Autodesk Inventor part; units mm, degrees
ref_plane "YZ Plane" through (0, 0, 0) normal (1, 0, 0) x (0, 1, 0)
ref_plane "XZ Plane" through (0, 0, 0) normal (0, 1, 0) x (-1, 0, 0)
ref_plane "XY Plane" through (0, 0, 0) normal (0, 0, 1) x (1, 0, 0)
sketch "Sketch1" plane through (0, 0, 0) normal (0, 0, 1) x (1, 0, 0)
  arc A0 (-220.016275, 220.016275) -> (-311.15, 0) centre (0, 0) ccw
  line L0 (-311.15, 0) -> (-304.8, 0)
  line L1 (0, 0) -> (-220.016275, 220.016275)
  line L2 (-311.15, 0) -> (0, 0)
extrude "Extrusion1" add sketch "Sketch1" along normal blind 3.175
sketch "Sketch4" plane through (0, 0, 0) normal (0, 0, -1) x (-1, 0, 0)
  arc A0 (311.15, 0) -> (220.016275, 220.016275) centre (0, 0) ccw
  line L0 (220.016275, 220.016275) -> (0, 0)
  line L1 (0, 0) -> (311.15, 0)
  arc A1 (301.625, 0) -> (213.281083, 213.281083) centre (0, 0) ccw
  arc A2 (303.2125, 0) -> (214.403615, 214.403615) centre (0, 0) ccw
  arc A3 (304.8, 0) -> (215.526147, 215.526147) centre (0, 0) ccw construction
  arc A4 (300.0375, 0) -> (212.158551, 212.158551) centre (0, 0) ccw construction
  circle A5 centre (215.526147, 215.526147) radius 1.5875
  circle A6 centre (212.158551, 212.158551) radius 1.5875
  circle A7 centre (233.490346, 195.921663) radius 1.5875
  circle A8 centre (229.84206, 192.860387) radius 1.5875
  circle A9 centre (249.677543, 174.826098) radius 1.5875
  circle A10 centre (245.776331, 172.09444) radius 1.5875
  circle A11 centre (263.964543, 152.4) radius 1.5875
  circle A12 centre (259.840097, 150.01875) radius 1.5875
  circle A13 centre (276.242613, 128.814046) radius 1.5875
  circle A14 centre (271.926323, 126.801327) radius 1.5875
  circle A15 centre (286.418311, 104.24774) radius 1.5875
  circle A16 centre (281.943025, 102.618869) radius 1.5875
  circle A17 centre (294.414192, 78.888045) radius 1.5875
  circle A18 centre (289.81397, 77.655419) radius 1.5875
  circle A19 centre (300.169403, 52.927965) radius 1.5875
  circle A20 centre (295.479256, 52.100965) radius 1.5875
  circle A21 centre (303.640144, 26.56507) radius 1.5875
  circle A22 centre (298.895767, 26.149991) radius 1.5875
  circle A23 centre (304.8, 0) radius 1.5875
  circle A24 centre (300.0375, 0) radius 1.5875
  circle A25 centre (219.969498, 210.989242) radius 1.5875
  circle A26 centre (304.733847, 6.35) radius 1.5875
  point P0 (231.058155, 193.880813)
  point P1 (232.274251, 194.901238)
  point P2 (247.076735, 173.004993)
  point P3 (248.377139, 173.915545)
  point P4 (261.214912, 150.8125)
  point P5 (262.589728, 151.60625)
  point P6 (273.365086, 127.472233)
  point P7 (274.80385, 128.14314)
  point P8 (283.434787, 103.161826)
  point P9 (284.926549, 103.704783)
  point P10 (291.347377, 78.066294)
  point P11 (292.880785, 78.47717)
  point P12 (297.042639, 52.376632)
  point P13 (298.606021, 52.652298)
  point P14 (300.477226, 26.288351)
  point P15 (302.058685, 26.426711)
  point P16 (301.625, 0)
  point P17 (303.2125, 0)
  dimension "d2" = 9.525
  dimension "d3" = 1.5875
  dimension "d4" = 1.5875
  dimension "d5" = 1.5875
  dimension "d8" = 45
  dimension "d10" = 6.35
  dimension "d13" = 3.175
  dimension "d14" = 6.35
sketch "Sketch4 outline for Extrusion2" plane through (0, 0, 0) normal (0, 0, -1) x (-1, 0, 0)
  circle A0 centre (233.490346, 195.921663) radius 1.5875
  circle A1 centre (249.677543, 174.826098) radius 1.5875
  circle A2 centre (263.964543, 152.4) radius 1.5875
  circle A3 centre (276.242613, 128.814046) radius 1.5875
  circle A4 centre (286.418311, 104.24774) radius 1.5875
  circle A5 centre (294.414192, 78.888045) radius 1.5875
  circle A6 centre (300.169403, 52.927965) radius 1.5875
  circle A7 centre (303.640144, 26.56507) radius 1.5875
  circle A8 centre (219.969498, 210.989242) radius 1.5875
  circle A9 centre (304.733847, 6.35) radius 1.5875
  circle A10 centre (229.84206, 192.860387) radius 1.5875
  circle A11 centre (245.776331, 172.09444) radius 1.5875
  circle A12 centre (259.840097, 150.01875) radius 1.5875
  circle A13 centre (271.926323, 126.801327) radius 1.5875
  circle A14 centre (281.943025, 102.618869) radius 1.5875
  circle A15 centre (289.81397, 77.655419) radius 1.5875
  circle A16 centre (295.479256, 52.100965) radius 1.5875
  circle A17 centre (298.895767, 26.149991) radius 1.5875
extrude "Extrusion2" cut sketch "Sketch4 outline for Extrusion2" against normal blind 25.4
sketch "Sketch7" plane through (0, 0, 3.175) normal (0, 0, 1) x (1, 0, 0)
  line L0 (-219.576555, 192.635787) -> (-45.990768, 19.05)
  line L1 (-45.990768, 19.05) -> (-291.478142, 19.05)
  arc A0 (-99.872305, 72.931537) -> (-122.190768, 19.05) centre (-45.990768, 19.05) ccw
  dimension "d29" = 152.4
extrude "Extrusion4" add sketch "Sketch7" against normal blind 3.175
sketch "Sketch9" plane through (0, 0, 3.175) normal (0, 0, 1) x (1, 0, 0)
  arc A0 (-220.016275, 220.016275) -> (-311.15, 0) centre (0, 0) ccw
  line L0 (0, 0) -> (-220.016275, 220.016275)
  arc A1 (-219.576555, 192.635787) -> (-291.478142, 19.05) centre (0, 0) ccw
  arc A2 (-201.574062, 174.633294) -> (-266.132217, 17.393478) centre (0, 0) ccw
  arc A3 (-181.389328, 159.133911) -> (-240.786292, 15.736957) centre (0, 0) ccw
  arc A4 (-162.295715, 142.382973) -> (-215.440366, 14.080435) centre (0, 0) ccw
  arc A5 (-143.202101, 125.632035) -> (-190.094441, 12.423913) centre (0, 0) ccw
  arc A6 (-124.108488, 108.881097) -> (-164.748515, 10.767391) centre (0, 0) ccw
  arc A7 (-105.014874, 92.130159) -> (-139.40259, 9.11087) centre (0, 0) ccw
  arc A8 (-66.827647, 58.628283) -> (-88.710739, 5.797826) centre (0, 0) ccw
  line L1 (-219.576555, 192.635787) -> (-201.574062, 174.633294)
  line L2 (-266.132217, 17.393478) -> (-291.478142, 19.05)
  line L3 (-215.440366, 14.080435) -> (-240.786292, 15.736957)
  line L4 (-88.710739, 5.797826) -> (-139.40259, 9.11087)
  line L5 (-164.748515, 10.767391) -> (-190.094441, 12.423913)
  line L6 (-66.827647, 58.628283) -> (-105.014874, 92.130159)
  line L7 (-143.202101, 125.632035) -> (-124.108488, 108.881097)
  line L8 (-181.389328, 159.133911) -> (-162.295715, 142.382973)
  dimension "d34" = 19.05
  dimension "d35" = 25.4
  dimension "d36" = 25.4
  dimension "d38" = 25.4
  dimension "d39" = 25.4
  dimension "d40" = 25.4
  dimension "d41" = 25.4
extrude "Extrusion5" cut sketch "Sketch9" against normal blind 3.175
properties part number "Side Panel" material "Polycarbonate, Clear"
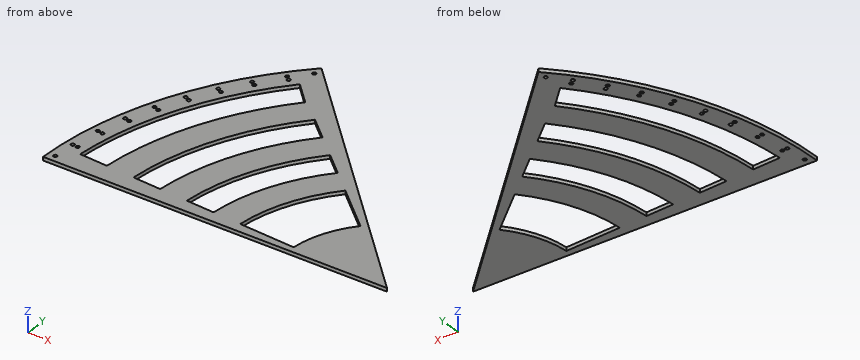
Verification items for the finished model (mm, model axes). Give positions to 0.01 mm unless a question says otherwise; leave off trailing zeros. Write each loop counter-clockwise with the first axis right and the second up, starting at its lowest first coordinate (ties: lowest second). Pieces come first, ordered by that corner, then holes. Notation, with made-up numbers: M 10.5,-27.75 L 34.5,-27.75 A11 cw 34.5,-12.75 Z; hole C 24.25,52 d11. An arc over 180 degrees is marked long. Put each result on its own line as item: value. Start each with the question number.
1. Scan lines: line 1 along X through (y, z) = (19.5, 1.1) (3 decimals); line 2 along X through (y, z) = (131.5, 1.35); line 3 along X through (y, z) = (59.5, 0.3). Record each from-to range of solid material in increasing order. Write a range as [from, to].
2. Section check D-D (y = 203). Record the cut outline in (x, z) (3 decimals).
3. Go/stop test with flat-tipped pins: pin 1 Ø2.5 at (x, y) = (-298.9, 26.15) entering from +Z; pin 2 Ø1 at (y, z) = (176, 0.5) entering from +X. Record where each tip stops, or that it passes through.
4. Section check C-C (z = 0.55). Give the number of separate pieces and of enclosed holes in the cut face, and give its area (3 significant figures).
5. Section check A-A (x = -72.5). Record the cut outline in (y, z) (3 decimals).
6. Section check B-B (y = 119). Record the cut outline in (x, z) (3 decimals).
Answer list:
1. line 1: [-310.538, -291.448], [-265.986, -240.511], [-215.018, -189.499], [-163.944, -138.332], [-86.735, -19.5]
1. line 2: [-282, -260.83], [-232.03, -202.32], [-171.23, -131.5]
1. line 3: [-305.41, -285.98], [-259.98, -233.85], [-207.54, -180.97], [-154.01, -126.4], [-67.82, -59.5]
2. outline: M -235.808,0 L -203,0 L -203,3.175 L -235.808,3.175 Z
3. pin 1: through
3. pin 2: x = -175.5
4. separate pieces: 1
4. enclosed holes: 22
4. area: 22,700 mm2
5. outline: M 0,0 L 51.449,0 L 51.449,3.175 L 0,3.175 Z; M 63.605,0 L 72.5,0 L 72.5,3.175 L 63.605,3.175 Z
6. outline: M -287.495,0 L -266.761,0 L -266.761,3.175 L -287.495,3.175 Z; M -238.679,0 L -209.916,0 L -209.916,3.175 L -238.679,3.175 Z; M -180.144,0 L -148.759,0 L -148.759,3.175 L -180.144,3.175 Z; M -135.643,0 L -119,0 L -119,3.175 L -135.643,3.175 Z
